Here's the drawing with two shaded views (mm, measured from the low corner). I have some questions. A direction names the side the tool comes from. Round coordinates to 2 decimals unless told otherwise and drop trailing zeros. Loops run counter-clockwise (first coordinate to the right, second up) from the corner with the lowest first, then second, coordinate; pieces in that order, holes last. Notation, with made-up numbers: (27, 20) -> (59, 20) arc R31 ccw to (59, 54) -> close; hole circle Ø3 at (71, -36). An arc over 180 degrees is marked (long way). Write item = value, one per line.
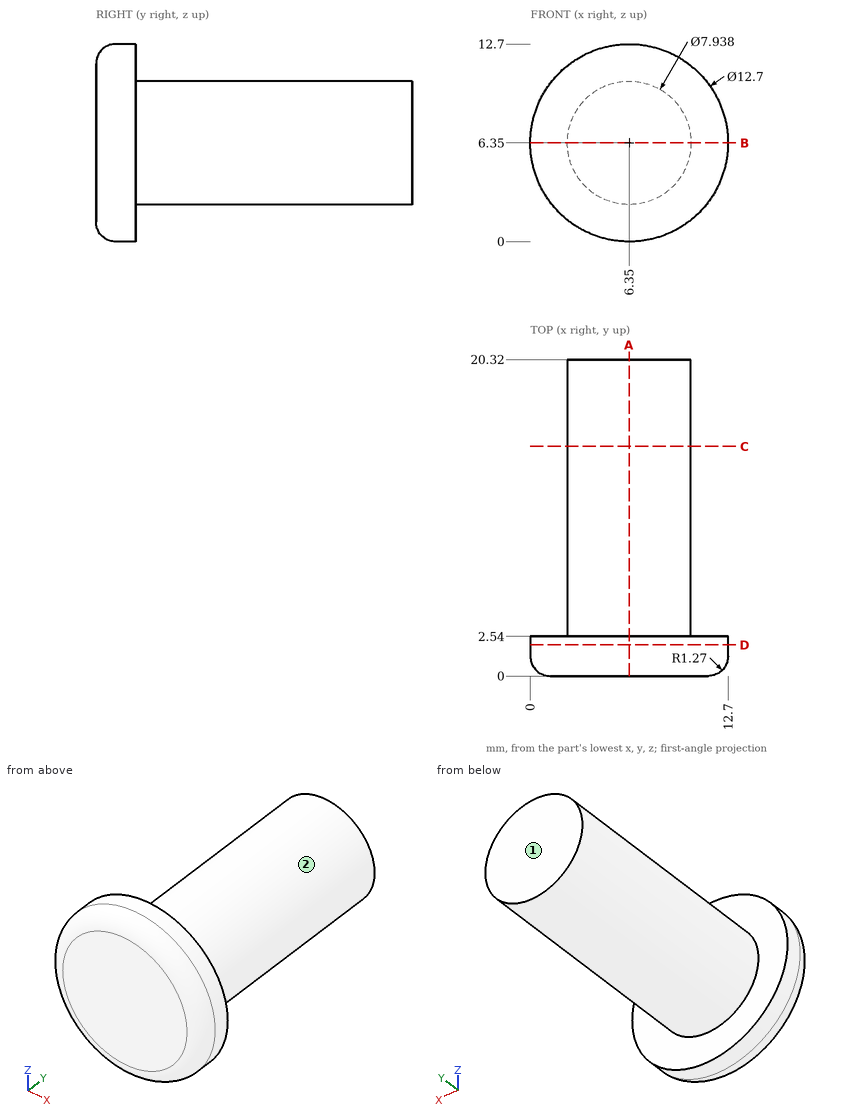
1. Suppose I cut it at A-A, the plane x = 6.35. List the corners of the cut face in (y, z) for me.
Entries:
outline = (0, 1.27) arc R1.27 ccw to (1.27, 0) -> (2.54, 0) -> (2.54, 2.38) -> (20.32, 2.38) -> (20.32, 10.32) -> (2.54, 10.32) -> (2.54, 12.7) -> (1.27, 12.7) arc R1.27 ccw to (0, 11.43) -> close
2. I'm going to push flat-ended pins straight in: pin 1 (6 mm diameter, centred on x = 8.5, y = 11.5, fed in from +Z); pin 2 (1.5 mm diameter, centred on y = 4.5, z = 8.5, fed in from +X); pin 3 (1 mm diameter, centred on x = 3.5, y = 17.5, fed in from +Z). Where does each tip first touch, or does it pass through?
Entries:
pin_1 = 10.32
pin_2 = 10.06
pin_3 = 9.55
3. For the marked faces 1 and 2, which set-ups out of +Z, -Z, +X, -X, +Y, -Y let a thin tool reach every point of the face, with its end or its side?
Entries:
face_1 = +Z, -Z, +X, -X, +Y
face_2 = +Y
4. Suppose I cut it at C-C, the plane y = 14.75. List the corners of the cut face in (x, z) for me.
Entries:
outline = circle Ø7.94 at (6.35, 6.35)
5. I need wall thicknesses on line 1 (Y direction, x = 10.25, z = 9.5); line 2 (Z direction, x = 6.5, y = 19.25) (1 decimal). Which ranges of each line are inside material? Lowest first, please. Write a range as [from, to].
Entries:
line_1 = [0, 2.54]
line_2 = [2.4, 10.3]
6. Suppose I cut it at D-D, the plane y = 2. List the corners of the cut face in (x, z) for me.
Entries:
outline = circle Ø12.7 at (6.35, 6.35)
7. Suppose I cut it at B-B, the plane z = 6.35. List the corners of the cut face in (x, y) for me, and give its area (3 significant figures).
Entries:
outline = (0, 1.27) arc R1.27 ccw to (1.27, 0) -> (11.43, 0) arc R1.27 ccw to (12.7, 1.27) -> (12.7, 2.54) -> (10.32, 2.54) -> (10.32, 20.32) -> (2.38, 20.32) -> (2.38, 2.54) -> (0, 2.54) -> close
area = 173 mm²
